Verification items for the finished model (mm, model axes). Face numbers are marked on the shaded views. A direction names the side the tool comes from. Coordinates: 2 decimals unless noted, no trailing zeros. Order: outer loops, then holes, each group sorted by start corner. A loop starts at its lowest first (then second) coordinate and runs counter-clockwise, first axis right, second up. Notation, with made-up numbers: M 37,17 L 96,17 A32 ccw 96,45 Z; hole C -11,74 d4. An arc over 180 degrees is marked long. Answer as a JSON object with one key per item and string values. Group by question number.
(1) Access from +Z, -Z, +X, -X, +Y, -Y to the whole of each face (thin tool, end or side, straight path). Record for the marked faces 4, 5 and 6.
(2) Mould release check, pull along Y, two halves, no side actions. Record for the marked faces 1, 2 and 3: released by +Y, released by -Y, zero draft, split by the parting line, or undercut.
(3) Cross-section at C-C (y = -42). Enter the section's corners in (x, z), plus the area to 3 significant figures.
(4) Material ranges on line 1 (Y direction, x = 10, z = 5.5); line 2 (X direction, y = -42, z = 11); line 3 (Z direction, x = 109.5, y = -16), recorded low to high.
(5) Gauge pin test, flat ends, axial feed: pin 1 Ø1.9 at (y, z) = (-24.5, 4.5) entering from -X; pin 2 Ø5 at (x, y) = (10, -8) entering from -Z; pin 3 Ø1 at (y, z) = (-9.5, 3.5) entering from +X; pin 4 Ø18.5 at (x, y) = (124, -25) entering from +Z. Record the tip position at first contact, or that the pin passes through.
(6) Cross-section at A-A (z = 7). Count the separate pieces of the cut face and the enclosed holes in it, plus the area to 3 significant figures.
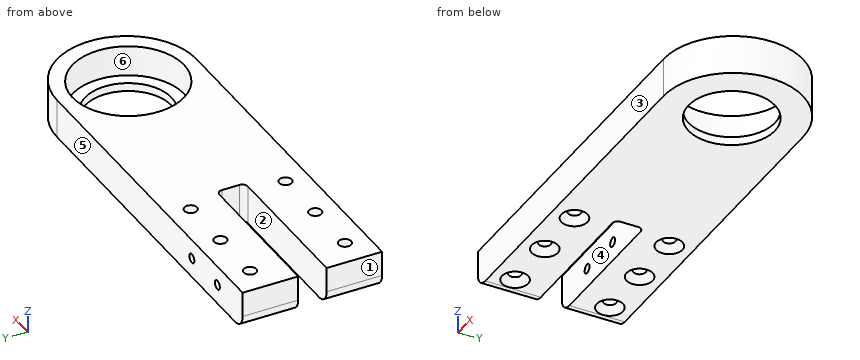
from build123d import *

# Parameters (mm, degrees)
BOSS_EXTRUDE1_DEPTH                             = 14
SKETCH2_W                                       = 55
SKETCH2_H                                       = 10.2
CUT_EXTRUDE1_DEPTH                              = 159.732479348
CSK_FOR_M4_FLAT_HEAD_MACHINE_SCREW1_D           = 4.5
CSK_FOR_M4_FLAT_HEAD_MACHINE_SCREW1_CSINK_D     = 9.4
CSK_FOR_M4_FLAT_HEAD_MACHINE_SCREW1_CSINK_ANGLE = 90
M4X0_7_TAPPED_HOLE1_D                           = 3.3
M4X0_7_TAPPED_HOLE1_DEPTH                       = 19.899999999
HOLE1_D                                         = 31.000000009
HOLE1_CBORE_D                                   = 40.00000001
HOLE1_CBORE_DEPTH                               = 11
FILLET1_R                                       = 2
FILLET2_R                                       = 5


with BuildPart() as part:
    # Sketch1 → Boss-Extrude1 (new body)
    with BuildSketch(Plane(origin=(0, 0, 0), x_dir=(-1, 0, 0), z_dir=(0, 0, -1))):
        with BuildLine():
            Line((0, 0), (-125, 0))
            ThreePointArc((-125, 0), (-150, -25), (-125, -50))
            Line((-125, -50), (0, -50))
            Line((0, -50), (0, 0))
        make_face()
    extrude(amount=-BOSS_EXTRUDE1_DEPTH)

    # Sketch2 → Cut-Extrude1 (cut, through all)
    with BuildSketch(Plane.XY.offset(14)):
        with Locations((27.5, -24.999999999)):
            Rectangle(SKETCH2_W, SKETCH2_H)
    extrude(amount=-CUT_EXTRUDE1_DEPTH, mode=Mode.SUBTRACT)

    # CSK for M4 Flat Head Machine Screw1 (through all)
    with Locations(Plane(origin=(0, 0, 0), x_dir=(-1, 0, 0), z_dir=(0, 0, -1))):
        with Locations((-10, -8), (-10, -42), (-30, -42), (-30, -8), (-50, -8), (-50, -42)):
            CounterSinkHole(CSK_FOR_M4_FLAT_HEAD_MACHINE_SCREW1_D / 2, CSK_FOR_M4_FLAT_HEAD_MACHINE_SCREW1_CSINK_D / 2, counter_sink_angle=CSK_FOR_M4_FLAT_HEAD_MACHINE_SCREW1_CSINK_ANGLE)

    # M4x0.7 Tapped Hole1
    with Locations(Plane(origin=(0, 0, 0), x_dir=(1, 0, 0), z_dir=(0, 1, 0))):
        with Locations((17, -7), (34.2, -7)):
            Hole(M4X0_7_TAPPED_HOLE1_D / 2, depth=M4X0_7_TAPPED_HOLE1_DEPTH)

    # Hole1 (through all)
    with Locations(Plane.XY.offset(14)):
        with Locations((123.999999995, -24.999999999)):
            CounterBoreHole(HOLE1_D / 2, HOLE1_CBORE_D / 2, HOLE1_CBORE_DEPTH)

    # Fillet1
    fillet1_edges = [part.edges().sort_by_distance(p)[0] for p in [
        (55, -19.899999999, 7),
        (55, -30.099999999, 7),
    ]]
    fillet(fillet1_edges, radius=FILLET1_R)

    # Fillet2
    fillet2_edges = [part.edges().sort_by_distance(p)[0] for p in [
        (0, -9.95, 0),
        (0, -40.05, 0),
    ]]
    fillet(fillet2_edges, radius=FILLET2_R)


solid = part.part
Taken from the geometry:
{
 "1": {"face 4": "+Z, -Z, -X", "face 5": "+Z, -Z, +X, -X, +Y", "face 6": "+Z"},
 "2": {"face 1": "zero draft", "face 2": "undercut", "face 3": "released by -Y"},
 "3": {"outline": "M 0,5 A5 ccw 5,0 L 5.3,0 L 7.75,2.45 L 7.75,14 L 0,14 Z; M 12.25,2.45 L 14.7,0 L 25.3,0 L 27.75,2.45 L 27.75,14 L 12.25,14 Z; M 32.25,2.45 L 34.7,0 L 45.3,0 L 47.75,2.45 L 47.75,14 L 32.25,14 Z; M 52.25,2.45 L 54.7,0 L 143.33,0 L 143.33,14 L 134.54,14 L 134.54,3 L 113.46,3 L 113.46,14 L 52.25,14 Z", "area": "1,560 mm²"},
 "4": {"line 1": "y = -50 to -44.25, -39.75 to -30.1, -19.9 to -10.25, -5.75 to 0", "line 2": "x = 0 to 7.75, 12.25 to 27.75, 32.25 to 47.75, 52.25 to 113.46, 134.54 to 143.33", "line 3": "z = 0 to 3"},
 "5": {"pin 1": "stops at x = 55", "pin 2": "stops at z = 2.2", "pin 3": "stops at x = 145", "pin 4": "passes through"},
 "6": {"separate pieces": "3", "enclosed holes": "7", "area": "5,190 mm²"}
}
